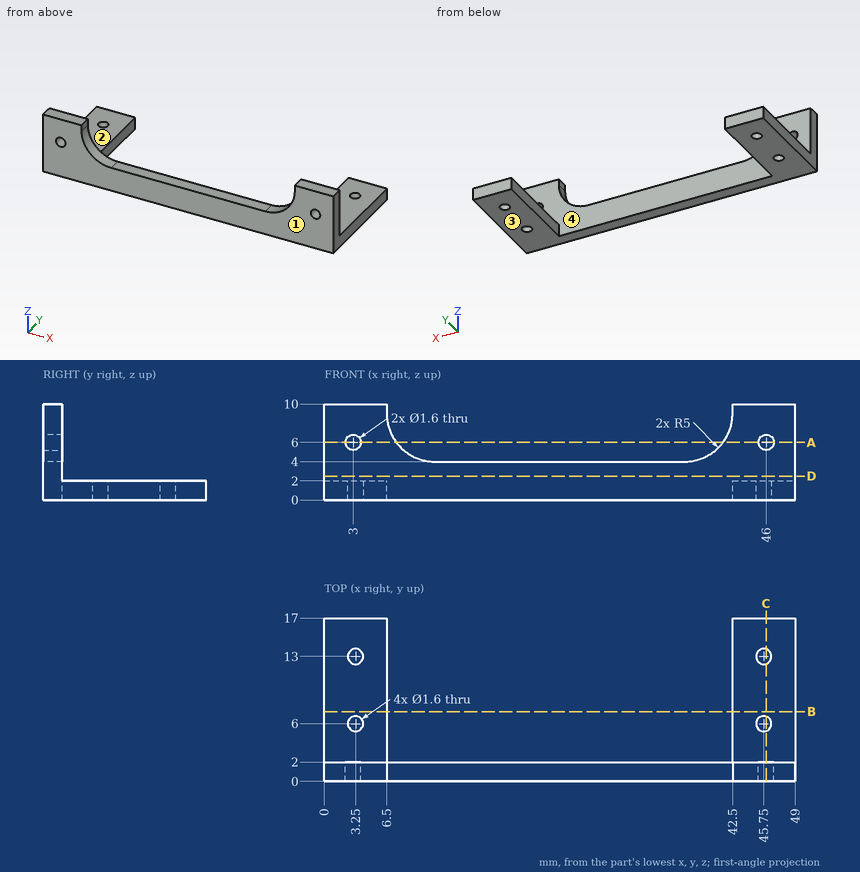
Geometry: see drawing. Coordinates: mm, zero at the bounding-box minimum. A direction names the side the tool comes from. Coordinates: 2 decimals unless noted, no trailing zeros. Order: outer loops, then holes, each group sorted by start corner. A loop starts at its lowest first (then second) coordinate and runs counter-clockwise, first axis right, second up. Notation, with made-up numbers: M 42,-16 L 67,-16 A25 cw 67,15 Z; hole C -27.5,-19.75 d5. An arc over 180 degrees is marked long. Write item = value, one per line. Start each with the question number.
(1) Line query: line 1 along Y through (x, z) = (45.75, 0.4); line 2 along Z through (x, y) = (46, 1.05); line 3 along X through (y, z) = (0.8, 6). Output: solid intervals per line, ascending. Write a range as [from, to].
(2) Section D-D on z = 2.5. Output: boundary loops of the cut face in (x, y).
(3) Section B-B on y = 7.25. Output: boundary loops of the cut face in (x, z).
(4) First-contact query: P1, Ø1, axis at x = 3, z = 6, coming from the -Y side; P2, Ø3, axis at x = 46.5, y = 10, coming from the +Z side; P3, Ø2, axis at x = 25, y = 0.5, coming from the +Z side; P4, Ø2, axis at x = 20, z = 2, coming from the +Y side. Flat tips, straight axial feed; report the tip coordinate or a pass-through.
(5) Section C-C on x = 46. Output: boundary loops of the cut face in (y, z).
(6) Reachability of the marked faces 1 and 2 from +Z, -Z, +X, -X, +Y, -Y: full face, straight path, thin tool, end or side. Return the list, or none.
(7) Pull-direction query (X, two-part tool) for the marked faces 3 and 4; classes: released by +X, released by -X, zero draft, split by the parting line, or undercut.
(8) Section A-A on z = 6. Output: boundary loops of the cut face in (x, y).
Result set:
q1.line_1 = [0, 5.2], [6.8, 12.2], [13.8, 17]
q1.line_2 = [0, 5.2], [6.8, 10]
q1.line_3 = [0, 2.2], [3.8, 7.5], [41.5, 45.2], [46.8, 49]
q2.outline = M 0,0 L 49,0 L 49,2 L 0,2 Z
q3.outline = M 0,0 L 6.5,0 L 6.5,2 L 0,2 Z; M 42.5,0 L 49,0 L 49,2 L 42.5,2 Z
q4.P1 = through
q4.P2 = 2
q4.P3 = 4
q4.P4 = 2
q5.outline = M 0,0 L 5.24,0 L 5.24,2 L 2,2 L 2,5.2 L 0,5.2 Z; M 0,6.8 L 2,6.8 L 2,10 L 0,10 Z; M 6.76,0 L 12.24,0 L 12.24,2 L 6.76,2 Z; M 13.76,0 L 17,0 L 17,2 L 13.76,2 Z
q6.face_1 = +Z, -Z, +X, -X, -Y
q6.face_2 = +Z, +X, -X, +Y
q7.face_3 = zero draft
q7.face_4 = undercut
q8.outline = M 0,0 L 2.2,0 L 2.2,2 L 0,2 Z; M 3.8,0 L 7.5,0 L 7.5,2 L 3.8,2 Z; M 41.5,0 L 45.2,0 L 45.2,2 L 41.5,2 Z; M 46.8,0 L 49,0 L 49,2 L 46.8,2 Z
